Build history of the part. All positions in model axes, mm. Face numbers are marked on the shaded views. A direction names the side the tool comes from. Round coordinates to 2 decimals unless told otherwise and drop trailing zeros. Order: outer loops, then holes, each group sorted by start corner. A loop starts at its lowest first (then second) coordinate and runs counter-clockwise, first axis right, second up. Notation, with made-up numbers: (-13, 79.5) -> (31, 79.5) arc R13 ccw to (31, 91.5) -> close; hole circle Ø4 at (27.5, -29). An arc over 180 degrees is marked (long way). Write item = value, one per line.
from build123d import *

# Parameters (mm, degrees)
SKETCH1_R           = 7.9375
BOSS_EXTRUDE1_DEPTH = 63.5
SKETCH4_R           = 5.5626
BOSS_EXTRUDE2_DEPTH = 38.1
SKETCH6_R           = 9.525
BOSS_EXTRUDE4_DEPTH = 38.1
SKETCH3_R           = 4.7625
CUT_EXTRUDE2_DEPTH  = 38.1


with BuildPart() as part:
    # Sketch1 → Boss-Extrude1 (new body)
    with BuildSketch(Plane.XY):
        Circle(SKETCH1_R)
    extrude(amount=BOSS_EXTRUDE1_DEPTH)

    # Sketch4 → Boss-Extrude2 (add)
    with BuildSketch(Plane(origin=(0, 0, 0), x_dir=(-1, 0, 0), z_dir=(0, 0, -1))):
        Circle(SKETCH4_R)
    extrude(amount=BOSS_EXTRUDE2_DEPTH)

    # Sketch6 → Boss-Extrude4 (add)
    with BuildSketch(Plane.XY.offset(12.7)):
        Circle(SKETCH6_R)
    extrude(amount=BOSS_EXTRUDE4_DEPTH)

    # Sketch3 → Cut-Extrude2 (cut)
    with BuildSketch(Plane.XY.offset(63.5)):
        Circle(SKETCH3_R)
    extrude(amount=-CUT_EXTRUDE2_DEPTH, mode=Mode.SUBTRACT)


solid = part.part
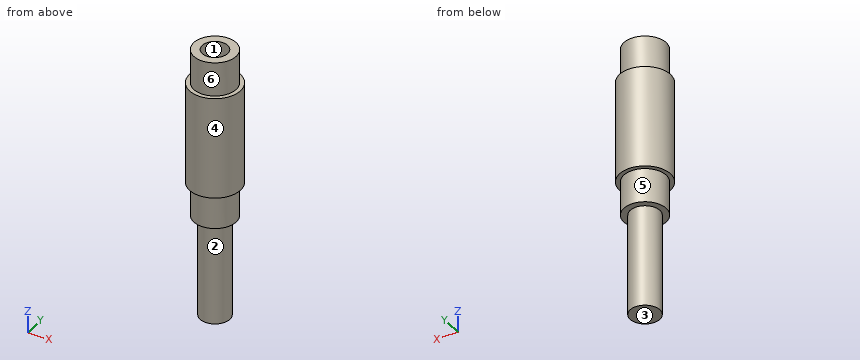
Q1. Probe probe 1 along Z at (x, y) = (-3.25, 0.5); probe 2 along Z at (x, y) = (1, 7.75); probe 3 along X at (y, z) = (-5.25, 49). List the from-to ranges inside material, lowest first.
Check values:
probe_1 = -38.1 to 25.4
probe_2 = 0 to 63.5
probe_3 = -7.95 to 7.95
Q2. Cut at D-D, the plane z = 4.5. List the corners of the cut face in (x, y) (1 decimal), and give its area (3 significant figures).
Check values:
outline = circle Ø15.9 at (0, 0)
area = 198 mm²
Q3. Cut at A-A, the plane y = 0. List the corners of the cut face in (x, z) (1 decimal), and give its area (3 significant figures).
Check values:
outline = (-9.5, 12.7) -> (-7.9, 12.7) -> (-7.9, 0) -> (-5.6, 0) -> (-5.6, -38.1) -> (5.6, -38.1) -> (5.6, 0) -> (7.9, 0) -> (7.9, 12.7) -> (9.5, 12.7) -> (9.5, 50.8) -> (7.9, 50.8) -> (7.9, 63.5) -> (4.8, 63.5) -> (4.8, 25.4) -> (-4.8, 25.4) -> (-4.8, 63.5) -> (-7.9, 63.5) -> (-7.9, 50.8) -> (-9.5, 50.8) -> close
area = 1,190 mm²
Q4. Cut at B-B, the plane x = 2. List the corners of the cut face in (y, z), and give its area (3 significant figures).
Check values:
outline = (-9.31, 12.7) -> (-7.68, 12.7) -> (-7.68, 0) -> (-5.19, 0) -> (-5.19, -38.1) -> (5.19, -38.1) -> (5.19, 0) -> (7.68, 0) -> (7.68, 12.7) -> (9.31, 12.7) -> (9.31, 50.8) -> (7.68, 50.8) -> (7.68, 63.5) -> (4.32, 63.5) -> (4.32, 25.4) -> (-4.32, 25.4) -> (-4.32, 63.5) -> (-7.68, 63.5) -> (-7.68, 50.8) -> (-9.31, 50.8) -> close
area = 1,170 mm²
Q5. Mould opens along X. For the marked faces 1, 2 and 3 say: released by +X, released by -X, zero draft, split by the parting line, or undercut.
Check values:
face_1 = undercut
face_2 = split by the parting line
face_3 = zero draft
Q6. Flat gauge pins, fed straight in: pin 1 (10 mm diameter, centred on y = -6, z = -12, fed in from -X); pin 2 (3 mm diameter, centred on x = 0.5, z = -10.5, fed in from -Y); pin 3 (2 mm diameter, centred on x = 2, z = 11.5, fed in from -Y). Where does each tip first touch, or does it go through?
Check values:
pin_1 = -5.47
pin_2 = -5.56
pin_3 = -7.87
Q7. Which spindle directions (+Z, -Z, +X, -X, +Y, -Y) get a long thin tool onto all of the face, cutting with end or side? Do the marked faces 4, 5 and 6. Say none if no direction does.
Check values:
face_4 = +Z, -Z
face_5 = -Z
face_6 = +Z
